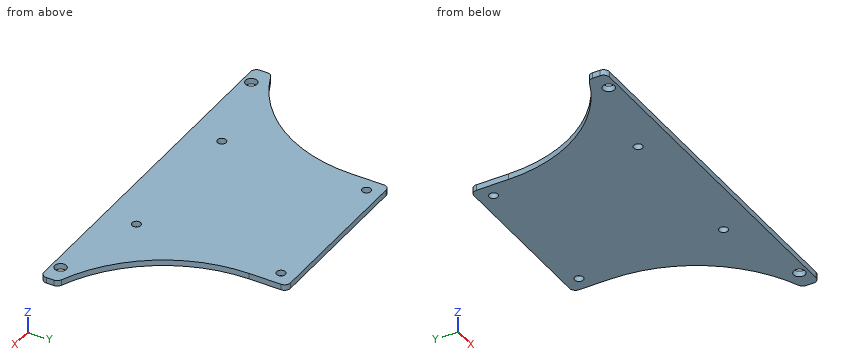
```python
from build123d import *

# Parameters (mm, degrees)
SKETCH_1_W      = 60
SKETCH_1_H      = 60
SKETCH_1_R      = 1.5
EXTRUDE_1_DEPTH = 2
SKETCH_2_W      = 125
SKETCH_2_H      = 6
SKETCH_2_R      = 2
EXTRUDE_2_DEPTH = 2
FILLET_1_R      = 50
FILLET_2_R      = 2


with BuildPart() as part:
    # 草图1 → 凸台-拉伸1 (new body)
    with BuildSketch(Plane.XY):
        with Locations((30, 30)):
            Rectangle(SKETCH_1_W, SKETCH_1_H)
        with Locations((5, 55)):
            Circle(SKETCH_1_R, mode=Mode.SUBTRACT)
        with Locations(Location((55, 55, 0), (0, 0, 180))):
            Circle(SKETCH_1_R, mode=Mode.SUBTRACT)
        with Locations((55, 5)):
            Circle(SKETCH_1_R, mode=Mode.SUBTRACT)
        with Locations(Location((5, 5, 0), (0, 0, 180))):
            Circle(SKETCH_1_R, mode=Mode.SUBTRACT)
    extrude(amount=EXTRUDE_1_DEPTH)

    # 草图2 → 凸台-拉伸2 (add)
    with BuildSketch(Plane.XY.offset(2)):
        with Locations((30, -3)):
            Rectangle(SKETCH_2_W, SKETCH_2_H)
        with Locations((-25.815, -3)):
            Circle(SKETCH_2_R, mode=Mode.SUBTRACT)
        with Locations(Location((85.815, -3, 0), (0, 0, 180))):
            Circle(SKETCH_2_R, mode=Mode.SUBTRACT)
    extrude(amount=-EXTRUDE_2_DEPTH)

    # 圆角1
    # the kernel refuses this fillet: 50 mm, written as the material it adds along each edge
    with BuildSketch(Plane(origin=(60, 0, 0), x_dir=(1, 0, 0), z_dir=(0, 0, 1))) as fillet_1_piece_1:
        with BuildLine():
            CenterArc((50, 46.837484988), FILLET_1_R, 180, 69.512684885)
            Line((0, 46.837484988), (-1, 46.837484988))
            Line((-1, 46.837484988), (-1, 0))
            Line((-1, 0), (0, -1))
            ThreePointArc((0, -1), (16.25, -1), (32.15, -0.9367497))
            Line((32.15, -0.9367497), (32.5, 0))
        make_face()
    extrude(amount=2)
    with BuildSketch(Plane(origin=(0, 0, 0), x_dir=(-1, 0, 0), z_dir=(0, 0, 1))) as fillet_1_piece_2:
        with BuildLine():
            CenterArc((50, -46.837484988), FILLET_1_R, 110.487315115, 69.512684885)
            Line((0, -46.837484988), (-1, -46.837484988))
            Line((-1, -46.837484988), (-1, 0))
            Line((-1, 0), (0, 1))
            ThreePointArc((0, 1), (16.25, 1), (32.15, 0.9367497))
            Line((32.15, 0.9367497), (32.5, 0))
        make_face()
    extrude(amount=2)

    # 圆角2
    fillet_2_edges = [part.edges().sort_by_distance(p)[0] for p in [
        (-32.5, -6, 1),
        (-32.5, 0, 1),
        (92.5, 0, 1),
        (92.5, -6, 1),
        (0, 60, 1),
        (60, 60, 1),
    ]]
    fillet(fillet_2_edges, radius=FILLET_2_R)


solid = part.part
```
The model under review builds one solid part; all positions refer to its coordinate system, in mm. Give positions to 0.01 mm unless a question says otherwise; leave off trailing zeros. Write each loop counter-clockwise with the first axis right and the second up, starting at its lowest first coordinate (ties: lowest second). Pieces come first, ordered by that corner, then holes. Notation, with made-up numbers: (73.25, -29.75) -> (91.25, -29.75) arc R34 cw to (91.25, 2.25) -> close; hole circle Ø8 at (-13, 42.5). An arc over 180 degrees is marked (long way). Answer in a Markdown table with one row per item.
1) Add section B-B on z = 1.6. State the section outline as (x, y) points (3 decimals).
Worked answers:
| item | result |
|---|---|
| outline | (-32.5, -4) arc R2 ccw to (-30.5, -6) -> (90.5, -6) arc R2 ccw to (92.5, -4) -> (92.5, -1.368) arc R2 ccw to (91.25, 0.486) arc R50 cw to (60, 46.837) -> (60, 58) arc R2 ccw to (58, 60) -> (2, 60) arc R2 ccw to (0, 58) -> (0, 46.837) arc R50 cw to (-31.25, 0.486) arc R2 ccw to (-32.5, -1.368) -> close; hole circle Ø4 at (-25.815, -3); hole circle Ø3 at (5, 5); hole circle Ø3 at (5, 55); hole circle Ø3 at (55, 5); hole circle Ø3 at (55, 55); hole circle Ø4 at (85.815, -3) |
2) Add section A-A on x = 55. State the section outline as (y, z) points, plus the area to 3 significant figures.
Worked answers:
| item | result |
|---|---|
| outline | (-6, 0) -> (3.5, 0) -> (3.5, 2) -> (-6, 2) -> close; (6.5, 0) -> (53.5, 0) -> (53.5, 2) -> (6.5, 2) -> close; (56.5, 0) -> (60, 0) -> (60, 2) -> (56.5, 2) -> close |
| area | 120 mm² |
3) Clearance check with flat-ended pins moving along their axes: P1, Ø2.5, axis at x = 55, y = 5, coming from the -Z side; P2, Ø0.6, axis at y = 51, z = 0.5, coming from the +X side. State where each tip first meets the part, or that it passes through.
Worked answers:
| item | result |
|---|---|
| P1 | through |
| P2 | x = 60 |
4) For L1, parallel to Y at x = 55, z = 0.5; L2, parallel to X at y = 47, z = 1.3; L3, parallel to X at y = 34, z = 1.65, list the stretches that pass through material, from the lowest coordinate up. Write a range as [from, to].
Worked answers:
| item | result |
|---|---|
| L1 | [-6, 3.5], [6.5, 53.5], [56.5, 60] |
| L2 | [0, 60] |
| L3 | [-1.68, 61.68] |
5) Add section D-D on x = -8. State the section outline as (y, z) points, plus the area to 3 significant figures.
Worked answers:
| item | result |
|---|---|
| outline | (-6, 0) -> (19.71, 0) -> (19.71, 2) -> (-6, 2) -> close |
| area | 51.4 mm² |
6) Add section C-C on y = 55. State the section outline as (x, z) points, plus the area to 3 significant figures.
Worked answers:
| item | result |
|---|---|
| outline | (0, 0) -> (3.5, 0) -> (3.5, 2) -> (0, 2) -> close; (6.5, 0) -> (53.5, 0) -> (53.5, 2) -> (6.5, 2) -> close; (56.5, 0) -> (60, 0) -> (60, 2) -> (56.5, 2) -> close |
| area | 108 mm² |
